```python
from build123d import *

# Parameters (mm, degrees)
SKETCH3_R                  = 8.172257435
SKETCH3_R_2                = 8.263232928
BOSS_EXTRUDE4_DEPTH        = 10
F_6_0_204_DIAMETER_HOLE1_D = 5.1816


with BuildPart() as part:
    # Sketch3 → Boss-Extrude4 (new body)
    # profile 1 of 5: a face of its own
    with BuildSketch(Plane.XY):
        Polygon((-49.555785737, 49.911142193), (-49.555785737, -49.688857807), (-6.690785737, -49.688857807), (-6.690785737, -42.753857807), (-6.690785737, -35.818857807), (0.244214263, -35.818857807), (7.179214263, -35.818857807), (7.179214263, -42.753857807), (7.179214263, -49.688857807), (50.044214263, -49.688857807), (50.044214263, 49.911142193), (7.179214263, 49.911142193), (7.179214263, 42.976142193), (7.179214263, 36.041142193), (0.244214299, 36.041142193), (-6.690785737, 36.041142193), (-6.690785737, 42.976142193), (-6.690785737, 49.911142193), align=None)
        with Locations((-11.1125, -22.225)):
            Circle(SKETCH3_R, mode=Mode.SUBTRACT)
        with Locations((11.1125, -22.225)):
            Circle(SKETCH3_R_2, mode=Mode.SUBTRACT)
    # profile 2 of 5: a face of its own
    with BuildSketch(Plane.XY):
        with BuildLine():
            Line((-6.690785737, -35.818857807), (-6.690785737, -42.753857807))
            ThreePointArc((-6.690785737, -42.753857807), (-4.659571264, -37.85007228), (0.244214263, -35.818857807))
            Line((0.244214263, -35.818857807), (-6.690785737, -35.818857807))
        make_face()
    # profile 3 of 5: a face of its own
    with BuildSketch(Plane.XY):
        with BuildLine():
            ThreePointArc((0.244214263, -35.818857807), (5.147999791, -37.85007228), (7.179214263, -42.753857807))
            Line((7.179214263, -42.753857807), (7.179214263, -35.818857807))
            Line((7.179214263, -35.818857807), (0.244214263, -35.818857807))
        make_face()
    # profile 4 of 5: a face of its own
    with BuildSketch(Plane.XY):
        with BuildLine():
            ThreePointArc((0.244214299, 36.041142193), (-4.659571252, 38.072356653), (-6.690785737, 42.976142193))
            Line((-6.690785737, 42.976142193), (-6.690785737, 36.041142193))
            Line((-6.690785737, 36.041142193), (0.244214299, 36.041142193))
        make_face()
    # profile 5 of 5: a face of its own
    with BuildSketch(Plane.XY):
        with BuildLine():
            Line((7.179214263, 36.041142193), (7.179214263, 42.976142193))
            ThreePointArc((7.179214263, 42.976142193), (5.147999803, 38.072356678), (0.244214299, 36.041142193))
            Line((0.244214299, 36.041142193), (7.179214263, 36.041142193))
        make_face()
    extrude(amount=BOSS_EXTRUDE4_DEPTH)

    # #6 (0.204) Diameter Hole1 (through all)
    with Locations(Plane(origin=(0, 0, 0), x_dir=(-1, 0, 0), z_dir=(0, 0, -1))):
        with Locations((44.205785737, -44.338857807), (-44.694214263, -44.338857807), (-44.694214263, 44.561142193), (44.205785737, 44.561142193), (44.205785737, 28.686142193), (44.205785737, -28.463857807), (-44.694214263, -28.463857807), (-44.694214263, 28.686142193)):
            Hole(F_6_0_204_DIAMETER_HOLE1_D / 2)


solid = part.part
```
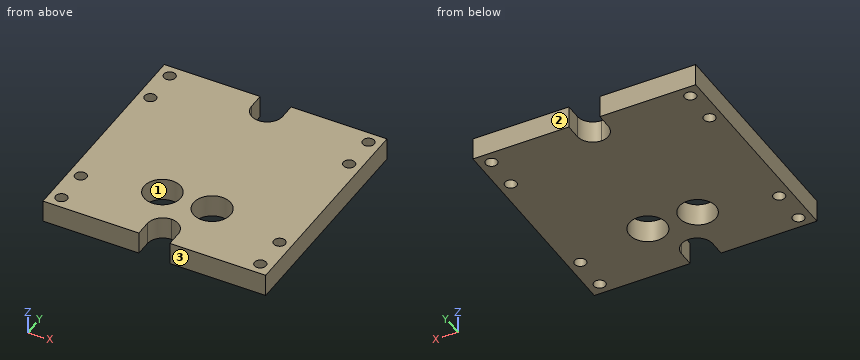
Build history of the part. All positions in model axes, mm. Face numbers are marked on the shaded views. Give positions to 0.01 mm unless a question says otherwise; leave off trailing zeros. Loops run counter-clockwise (first coordinate to the right, second up) from the corner with the lowest first, then second, coordinate; pieces in that order, holes last. Notation, with made-up numbers: (47.25, 54.5) -> (52.25, 54.5) arc R20 cw to (52.25, 67.5) -> close; hole circle Ø8 at (26.5, 39). An arc over 180 degrees is marked (long way). One line per question, with ' | ' between items. Start each with the question number.
1) Cut at D-D (y = -16). Give the cut face in (x, z).
2) Cut at B-B (y = -38.5). Give the cut face in (x, z).
3) Cut at A-A (x = -12.5). Give the cut face in (y, z).
4) Probe L1, parallel to X at y = -22, z = 8; L2, parallel to X at y = -44, z = 7.75; L3, parallel to X at y = -19.5, z = 9.5. List the from-to ranges inside material, lowest first.
5) Cut at C-C (z = 5). Count the separate pieces of the cut face and the enclosed holes in it, plus the area to 3 significant figures.
6) Two-plate mould, pull along Y, no slides. Class the marked faces 1, 2 and 3: released by +Y, released by -Y, zero draft, split by the parting line, or undercut.
Return value:
1) outline: (-49.56, 0) -> (-16.41, 0) -> (-16.41, 10) -> (-49.56, 10) -> close; (-5.82, 0) -> (5.68, 0) -> (5.68, 10) -> (-5.82, 10) -> close; (16.55, 0) -> (50.04, 0) -> (50.04, 10) -> (16.55, 10) -> close
2) outline: (-49.56, 0) -> (-5.23, 0) -> (-5.23, 10) -> (-49.56, 10) -> close; (5.72, 0) -> (50.04, 0) -> (50.04, 10) -> (5.72, 10) -> close
3) outline: (-49.69, 0) -> (-30.28, 0) -> (-30.28, 10) -> (-49.69, 10) -> close; (-14.17, 0) -> (49.91, 0) -> (49.91, 10) -> (-14.17, 10) -> close
4) L1: -49.56 to -19.28, -2.94 to 2.85, 19.37 to 50.04 | L2: -49.56 to -46.77, -41.64 to -6.69, 7.18 to 42.13, 47.26 to 50.04 | L3: -49.56 to -18.82, -3.41 to 3.31, 18.91 to 50.04
5) separate pieces: 1 | enclosed holes: 10 | area: 8,980 mm^2
6) face 1: undercut | face 2: released by +Y | face 3: released by -Y
